Could you check a few things on this model? Use its own coordinates, in mm. Face numbers are marked on the shaded views. A direction names the side the tool comes from. Round coordinates to 2 decimals unless told otherwise and drop trailing zeros. Write each loop counter-clockwise with the first axis right and the second up, starting at its lowest first coordinate (ties: lowest second). Pieces come first, ordered by that corner, then holes. Notation, with made-up numbers: (-36, 83) - (-4, 83) arc R22 cw to (-4, 94) - close; hole circle Ø10 at (39.25, 21). An arc over 180 degrees is marked (long way). Put each result on its own line as item: value.
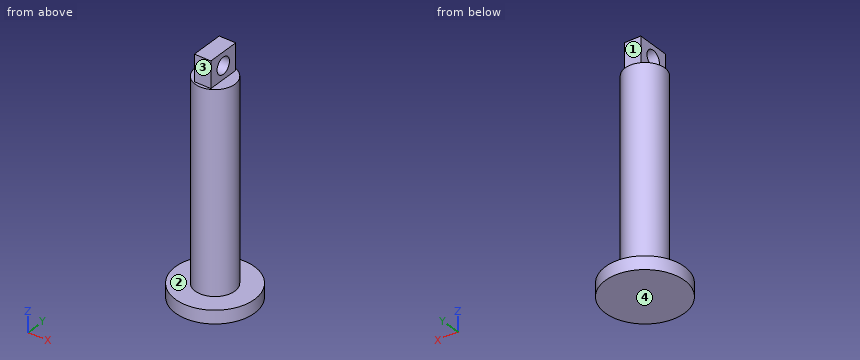
from build123d import *

# Parameters (mm, degrees)
SKETCH1_R           = 6
BOSS_EXTRUDE1_DEPTH = 2
SKETCH2_R           = 3
BOSS_EXTRUDE2_DEPTH = 30
SKETCH3_W           = 2.5
SKETCH3_H           = 5
BOSS_EXTRUDE3_DEPTH = 4
CUT_EXTRUDE1_REACH  = 39.21
SKETCH4_R           = 1.25


with BuildPart() as part:
    # Sketch1 → Boss-Extrude1 (new body)
    with BuildSketch(Plane.XY):
        Circle(SKETCH1_R)
    extrude(amount=BOSS_EXTRUDE1_DEPTH)

    # Sketch2 → Boss-Extrude2 (add)
    with BuildSketch(Plane.XY.offset(2)):
        Circle(SKETCH2_R)
    extrude(amount=BOSS_EXTRUDE2_DEPTH)

    # Sketch3 → Boss-Extrude3 (add)
    with BuildSketch(Plane.XY.offset(32)):
        Rectangle(SKETCH3_W, SKETCH3_H)
    extrude(amount=BOSS_EXTRUDE3_DEPTH)

    # Sketch4 → Cut-Extrude1 (cut, up to next)
    with BuildSketch(Plane.ZY.offset(1.25), mode=Mode.PRIVATE) as cut_extrude1_sk1:
        with Locations((34, 0)):
            Circle(SKETCH4_R)
    cut_extrude1_tool1 = extrude(cut_extrude1_sk1.sketch, amount=-CUT_EXTRUDE1_REACH, mode=Mode.PRIVATE) & part.part
    add(cut_extrude1_tool1.solids().sort_by_distance((-1.25, 0, 34))[0], mode=Mode.SUBTRACT)


solid = part.part
(1) I'm going to push flat-ended pins straight in: pin 1 (1.2 mm diameter, centred on y = -1, z = 34, fed in from +X); pin 2 (2 mm diameter, centred on y = -1, z = 33.5, fed in from -X); pin 3 (0.8 mm diameter, centred on x = 0.5, z = 34, fed in from +Y). Where does each tip first touch, or does it pass through?
Values found:
pin 1: stops at x = 1.25
pin 2: stops at x = -1.25
pin 3: stops at y = 2.5
(2) Imagine slicing it at C-C, the plane x = 2. List the corners of the cut face in (y, z) for me.
Values found:
outline: (-5.66, 0) - (5.66, 0) - (5.66, 2) - (2.24, 2) - (2.24, 32) - (-2.24, 32) - (-2.24, 2) - (-5.66, 2) - close
(3) Imagine slicing it at B-B, the plane y = 0. List the corners of the cut face in (x, z) for me.
Values found:
outline: (-6, 0) - (6, 0) - (6, 2) - (3, 2) - (3, 32) - (1.25, 32) - (1.25, 32.75) - (-1.25, 32.75) - (-1.25, 32) - (-3, 32) - (-3, 2) - (-6, 2) - close; (-1.25, 35.25) - (1.25, 35.25) - (1.25, 36) - (-1.25, 36) - close
(4) Imagine slicing it at A-A, the plane z = 34. List the corners of the cut face in (x, y) for me, then the cut area to 3 significant figures.
Values found:
outline: (-1.25, -2.5) - (1.25, -2.5) - (1.25, -1.25) - (-1.25, -1.25) - close; (-1.25, 1.25) - (1.25, 1.25) - (1.25, 2.5) - (-1.25, 2.5) - close
area: 6.25 mm^2
(5) Please list where these lines run through material, in increasing order: probe 1 along Z at (x, y) = (0, -3.5); probe 2 along X at (y, z) = (-2.75, 26); probe 3 along Y at (x, z) = (-1, 31). Write a range as from..to.
Values found:
probe 1: z = 0..2
probe 2: x = -1.2..1.2
probe 3: y = -2.83..2.83
(6) For the marked faces 1, 2, 3 and 4, which set-ups out of +Z, -Z, +X, -X, +Y, -Y let a thin tool reach every point of the face, with its end or its side?
Values found:
face 1: +Z, +X, -X, +Y
face 2: +Z
face 3: +Z, +X, -X, -Y
face 4: -Z, +X, -X, +Y, -Y
(7) Imagine slicing it at D-D, the plane y = 2. List the corners of the cut face in (x, z) for me, then the cut area to 3 significant figures.
Values found:
outline: (-5.66, 0) - (5.66, 0) - (5.66, 2) - (2.24, 2) - (2.24, 32) - (1.25, 32) - (1.25, 36) - (-1.25, 36) - (-1.25, 32) - (-2.24, 32) - (-2.24, 2) - (-5.66, 2) - close
area: 167 mm^2
